Work out the finished part from the listing and answer in its coordinate system (mm). A direction names the side the tool comes from. Round coordinates to 2 decimals unless told otherwise and drop trailing zeros. Loops run counter-clockwise (first coordinate to the right, second up) from the corner with the lowest first, then second, coordinate; pieces in that order, holes last. Notation, with made-up numbers: (30, 35.5) -> (34, 35.5) arc R6 ccw to (34, 40.5) -> close; hole circle Ø10 at (52, 57.5). An arc over 180 degrees is marked (long way). Write item = value, one per line. Start each with the question number.
Autodesk Inventor part; units mm, degrees
ref_plane "YZ Plane" through (0, 0, 0) normal (1, 0, 0) x (0, 1, 0)
ref_plane "XZ Plane" through (0, 0, 0) normal (0, 1, 0) x (-1, 0, 0)
ref_plane "XY Plane" through (0, 0, 0) normal (0, 0, 1) x (1, 0, 0)
sketch "Sketch1" plane through (0, 0, 0) normal (0, 0, 1) x (1, 0, 0)
  line L0 (-6.3366, 6.9163) -> (21.6034, 6.9163)
  line L1 (21.6034, 6.9163) -> (21.6034, -8.3237)
  line L2 (21.6034, -8.3237) -> (-6.3366, -8.3237)
  line L3 (-6.3366, -8.3237) -> (-6.3366, 6.9163)
  point P0 (0, 0)
  dimension "d0" = 27.94
  dimension "d1" = 15.24
extrude "Extrusion1" add sketch "Sketch1" along normal blind 7.62
sketch "Sketch2" plane through (0, 0, 7.62) normal (0, 0, 1) x (1, 0, 0)
  line L0 (-6.3366, 6.9163) -> (-6.3366, -8.3237)
  line L1 (21.6034, -8.3237) -> (21.6034, 6.9163)
  line L2 (21.6034, -0.052) -> (21.6034, 2.361)
  line L3 (-6.3366, 2.361) -> (-6.3366, -0.052)
  line L4 (21.6034, 6.9163) -> (-6.3366, 6.9163)
  line L5 (-6.3366, -8.3237) -> (21.6034, -8.3237)
  line L6 (0.9631, 2.361) -> (-0.2406, 2.361)
  line L7 (-0.2406, -0.052) -> (0.9631, -0.052)
  line L8 (-0.2406, -0.052) -> (-0.2406, 2.361)
  line L9 (-0.2406, -0.052) -> (3.0821, -0.052)
  line L10 (3.0821, -0.052) -> (3.0821, 2.361)
  line L11 (3.0821, 2.361) -> (-0.2406, 2.361)
  line L12 (-0.2406, 2.361) -> (-0.2406, -0.052)
  line L13 (14.3038, 2.361) -> (15.5074, 2.361)
  line L14 (15.5074, -0.052) -> (14.3038, -0.052)
  line L15 (15.5074, -0.052) -> (15.5074, 2.361)
  line L16 (15.5074, -0.052) -> (12.1847, -0.052)
  line L17 (12.1847, -0.052) -> (12.1847, 2.361)
  line L18 (12.1847, 2.361) -> (15.5074, 2.361)
  line L19 (15.5074, 2.361) -> (15.5074, -0.052)
  line L20 (-6.3366, -0.7037) -> (21.6034, -0.7037)
  line L21 (-6.3366, 2.361) -> (21.6034, 2.361)
  line L22 (21.6034, 2.361) -> (21.6034, -0.052)
  line L23 (21.6034, -0.052) -> (-6.3366, -0.052)
  line L24 (-6.3366, -0.052) -> (-6.3366, 2.361)
  point P0 (0, 0)
  point P1 (-0.2406, 1.1545)
  point P2 (15.2669, -0.3643)
  point P3 (15.5074, 1.1545)
  point P4 (15.5074, -0.052)
  point P5 (21.6034, -0.052)
  point P6 (15.5074, 2.361)
  point P7 (-6.3366, -0.052)
  point P8 (-0.2406, -0.052)
  point P9 (-0.2406, 2.361)
  point P10 (-6.3366, 2.361)
  point P11 (3.0821, -0.052)
  point P12 (12.1847, -0.052)
  point P13 (12.1847, 2.361)
  point P14 (3.0821, 2.361)
  dimension "d6" = 6.096
extrude "Extrusion2" add sketch "Sketch2" along normal blind 8.7376 contours L6 L11 L10 L9 L7 L8 | L15 L14 L16 L17 L18 L13
sketch "Sketch3" plane through (-0.2406, 2.361, 7.62) normal (0, 1, 0) x (1, 0, 0)
  line L0 (3.3227, -8.7376) -> (0, -8.7376)
  line L1 (-6.096, 7.62) -> (21.844, 7.62)
  line L2 (3.3227, -11.3552) -> (3.3227, -8.7376)
  line L3 (12.4253, -11.3552) -> (12.4253, -8.7376)
  line L4 (17.2091, -8.255) -> (17.2091, -15.2732)
  line L5 (17.2091, -15.2732) -> (14.9854, -19.057)
  line L6 (14.9854, -19.057) -> (12.4253, -19.057)
  line L7 (12.4253, -19.057) -> (12.4253, -8.7376)
  line L8 (7.874, 7.62) -> (7.874, -24.8322)
  line L9 (3.3227, -11.3552) -> (3.3227, -8.7376)
  line L10 (-1.4611, -8.255) -> (-1.4611, -15.2732)
  line L11 (-1.4611, -15.2732) -> (0.7626, -19.057)
  line L12 (0.7626, -19.057) -> (3.3227, -19.057)
  line L13 (3.3227, -19.057) -> (3.3227, -8.7376)
  line L14 (17.2091, -8.255) -> (12.4253, -8.255)
  line L15 (12.4253, 0) -> (12.4253, -8.7376)
  line L16 (12.4253, -8.255) -> (12.4253, -8.7376)
  line L17 (-1.4611, -8.255) -> (3.3227, -8.255)
  line L18 (3.3227, 0) -> (3.3227, -8.7376)
  line L19 (3.3227, -8.255) -> (3.3227, -8.7376)
  point P0 (0.2406, 7.62)
extrude "Extrusion4" add sketch "Sketch2" along normal blind 25.4 contours L6 L11 L10 L9 L7 L8 | L15 L14 L16 L17 L18 L13
sketch "Sketch4" plane through (-6.3366, 6.9163, 0) normal (0, 1, 0) x (1, 0, 0)
  point P0 (6.3366, 0)
sketch "Sketch5" plane through (0, 0, 7.62) normal (0, 0, 1) x (1, 0, 0)
  line L0 (21.6034, 6.9163) -> (-6.3366, 6.9163)
  line L1 (-6.3366, 15.6735) -> (21.6034, 15.6735)
  line L2 (21.6034, 15.6735) -> (21.6034, 6.9163)
  line L3 (21.6034, 6.9163) -> (-6.3366, 6.9163)
  line L4 (-6.3366, 6.9163) -> (-6.3366, 15.6735)
  point P0 (0, 0)
extrude "Extrusion5" add sketch "Sketch5" along normal blind 17.145 and the other way blind 7.62
extrude "Extrusion6" cut sketch "Sketch2" against normal blind 25.4 contours L20 L1 L5 L0
extrude "Extrusion7" add sketch "Sketch2" along normal blind 4.7625 contours L21 L8 L23 L0 | L1 L23 L15 L21 | L21 L17 L23 L10
extrude "Extrusion8" add sketch "Sketch3" against normal up to surface (2.413 mm away)
sketch "Sketch6" plane through (-6.3366, -0.052, 7.62) normal (0, -1, 0) x (1, 0, 0)
  line L0 (27.94, 0) -> (27.94, 4.7625)
  line L1 (21.844, 4.7625) -> (21.844, 8.255)
  line L2 (27.94, 0) -> (21.844, 0)
  line L3 (21.844, 0) -> (21.844, 4.7625)
  line L4 (21.844, 4.7625) -> (27.94, 4.7625)
  line L5 (27.94, 4.7625) -> (27.94, 0)
  line L6 (18.5213, 4.7625) -> (18.5213, 25.4)
  line L7 (18.5213, 4.7625) -> (9.4187, 4.7625)
  line L8 (9.4187, 4.7625) -> (9.4187, 0)
  line L9 (9.4187, 0) -> (18.5213, 0)
  line L10 (18.5213, 0) -> (18.5213, 4.7625)
  line L11 (6.096, 4.7625) -> (6.096, 8.255)
  line L12 (0, 0) -> (0, 4.7625)
  line L13 (6.096, 4.7625) -> (0, 4.7625)
  line L14 (0, 4.7625) -> (0, 0)
  line L15 (0, 0) -> (6.096, 0)
  line L16 (6.096, 0) -> (6.096, 4.7625)
  point P0 (6.3366, -7.62)
  point P1 (21.844, 8.7376)
  point P2 (18.5213, 19.057)
  point P3 (6.096, 8.7376)
extrude "Extrusion9" cut sketch "Sketch6" against normal up to surface (6.9683 mm away)
sketch "Sketch7" plane through (12.1847, -0.052, 7.62) normal (0, -1, 0) x (1, 0, 0)
  line L0 (3.3227, 17.7594) -> (4.7838, 15.2732)
  line L1 (3.3227, 17.7594) -> (2.3659, 19.3874)
  line L2 (2.3659, 19.3874) -> (2.3659, 25.4)
  line L3 (3.3227, 25.4) -> (0, 25.4)
  line L4 (3.3227, 17.7594) -> (3.3227, 25.4)
  line L5 (2.3659, 25.4) -> (3.3227, 25.4)
  line L6 (3.3227, 25.4) -> (3.3227, 17.7594)
  line L7 (-18.5213, -7.62) -> (9.4187, -7.62)
  line L8 (-12.4253, 17.7594) -> (-11.4685, 19.3874)
  line L9 (-11.4685, 19.3874) -> (-11.4685, 25.4)
  line L10 (-12.4253, 17.7594) -> (-12.4253, 25.4)
  line L11 (-11.4685, 25.4) -> (-12.4253, 25.4)
  line L12 (-12.4253, 25.4) -> (-12.4253, 17.7594)
  line L13 (-12.4253, 8.7376) -> (-13.8865, 8.255)
  line L14 (-9.1825, 8.7376) -> (-9.1026, 8.7376)
  line L15 (-9.1026, 0) -> (-9.1026, 25.4)
  line L16 (-10.6842, 5.3569) -> (-10.764, 0)
  line L17 (-9.1026, 0) -> (-12.4253, 0)
  line L18 (-9.1026, 0) -> (-9.1026, 8.7376)
  line L19 (-10.764, 0) -> (-9.1026, 0)
  line L20 (9.4187, -7.62) -> (-18.5213, -7.62)
  line L21 (-18.5213, 17.145) -> (9.4187, 17.145)
  line L22 (1.5816, 5.3569) -> (1.6613, 0)
  line L23 (1.6613, 0) -> (0, 0)
  line L24 (0, 0) -> (0, 8.7376)
  line L25 (-4.5513, -7.62) -> (-4.5513, 0)
  line L26 (-4.5513, 11.274) -> (-4.5513, 11.3382)
  line L27 (-9.1026, 8.7376) -> (-10.6842, 5.3569)
  line L28 (0, 8.7376) -> (1.5816, 5.3569)
  point P0 (-12.1847, -7.62)
extrude "Extrusion10" cut sketch "Sketch7" against normal up to surface (6.9683 mm away)
fillet "Fillet1" radius 3.175 4 edges at (0.7162, 1.1545, 33.02) (14.5507, 1.1545, 33.02) (16.9686, 1.1545, 22.8932) (-1.7017, 1.1545, 22.8932)
sketch "Sketch8" plane through (-0.2406, -0.052, 7.62) normal (0, -1, 0) x (1, 0, 0)
  arc A0 (-1.0234, 16.018) -> (-1.4611, 14.4093) centre (1.7139, 14.4093) ccw
  line L0 (-1.4611, 8.255) -> (-1.4611, 14.4093)
  line L1 (0, 0) -> (0, 8.255)
  line L2 (1.6613, 0) -> (0, 0)
  line L3 (1.6613, 0) -> (1.7411, 5.3569)
  line L4 (1.7411, 5.3569) -> (3.3227, 8.7376)
  line L5 (3.3227, 8.7376) -> (3.3227, 25.4)
  arc A1 (3.3227, 25.4) -> (0.9568, 22.3298) centre (4.1318, 22.3298) ccw
  line L6 (0.9568, 22.3298) -> (0.9568, 19.3874)
  line L7 (0.9568, 19.3874) -> (-1.0234, 16.018)
  arc A2 (17.2091, 14.4093) -> (16.7714, 16.018) centre (14.0341, 14.4093) ccw
  line L8 (16.7714, 16.018) -> (14.7912, 19.3874)
  line L9 (14.7912, 19.3874) -> (14.7912, 22.3298)
  arc A3 (14.7912, 22.3298) -> (12.4253, 25.4) centre (11.6162, 22.3298) ccw
  line L10 (12.4253, 8.7376) -> (12.4253, 25.4)
  line L11 (12.4253, 8.7376) -> (14.0069, 5.3569)
  line L12 (14.0069, 5.3569) -> (14.0867, 0)
  line L13 (15.748, 0) -> (14.0867, 0)
  line L14 (15.748, 0) -> (15.748, 8.255)
  line L15 (17.2091, 14.4093) -> (17.2091, 8.255)
  line L16 (17.2091, 8.255) -> (15.748, 8.255)
  line L17 (0, 8.255) -> (-1.4611, 8.255)
  point P0 (0.2406, -7.62)
extrude "Extrusion11" add sketch "Sketch8" against normal blind 3.81
sketch "Sketch9" plane through (0, 0, 7.62) normal (0, 0, 1) x (1, 0, 0)
  line L0 (9.6447, 0.3123) -> (5.6221, 0.3123)
  line L1 (5.6221, 0.3123) -> (5.6221, 4.1223)
  line L2 (5.6221, 4.1223) -> (9.6447, 4.1223)
  line L3 (9.6447, 4.1223) -> (9.6447, 0.3123)
  line L4 (12.1847, -0.052) -> (12.1847, 3.758)
  line L5 (3.0821, -0.052) -> (3.0821, 3.758)
  point P0 (0, 0)
  dimension "d30" = 2.54
  dimension "d31" = 2.54
extrude "Extrusion12" add sketch "Sketch9" along normal blind 18.0975
sketch "Sketch10" plane through (21.6034, 6.9163, 24.765) normal (1, 0, 0) x (0, 0, -1)
  line L0 (17.145, 0) -> (0, 0)
  line L1 (24.765, -7.62) -> (17.145, -7.62)
  line L2 (17.145, 0) -> (24.765, 0)
  line L3 (24.765, 0) -> (24.765, -7.62)
  line L4 (24.765, -7.62) -> (17.145, -7.62)
  line L5 (17.145, -7.62) -> (17.145, 0)
  point P0 (24.765, -6.9163)
extrude "Extrusion13" add sketch "Sketch10" along normal blind 6.1214 and the other way blind 34.0614
sketch "Sketch11" plane through (0, 0, 7.62) normal (0, 0, 1) x (1, 0, 0)
  line L0 (21.6034, 15.6735) -> (-6.3366, 15.6735)
  line L1 (9.6447, 0.3123) -> (5.6221, 0.3123)
  line L2 (-12.458, -0.7037) -> (-12.458, 6.9163)
  line L3 (-12.458, -0.7037) -> (27.7248, -0.7037)
  line L4 (-11.1046, -0.7037) -> (-12.458, -0.7037)
  line L5 (-12.458, -0.7037) -> (-12.458, 4.1961)
  line L6 (21.6034, -0.7037) -> (27.7131, -0.7037)
  line L7 (27.7131, -0.7037) -> (27.7131, 4.8182)
  line L8 (27.7131, 4.8182) -> (22.941, 4.8182)
  line L9 (21.6034, 4.8182) -> (21.6034, -0.7037)
  line L10 (-6.3366, -0.7037) -> (-12.4462, -0.7037)
  line L11 (-12.4462, -0.7037) -> (-12.4462, 4.8182)
  line L12 (-12.4462, 4.8182) -> (-7.6742, 4.8182)
  line L13 (-6.3366, 4.8182) -> (-6.3366, -0.7037)
  line L14 (21.6034, 6.9163) -> (27.7248, 6.9163)
  line L15 (22.941, 4.8182) -> (22.941, -0.7037)
  line L16 (7.6334, 0.3123) -> (7.6334, -0.7037)
  line L17 (-7.6742, 4.8182) -> (-7.6742, -0.7037)
  point P0 (0, 0)
  point P1 (22.941, 6.9163)
  point P2 (-7.6742, 6.9163)
  point P3 (-7.6742, -0.7037)
extrude "Extrusion14" add sketch "Sketch11" along normal blind 15.875
properties part number "Attachment6"
Item 1: Section B-B (x = 7.5) is taken. Determine the outline of the cut face in (y, z) (1 decimal), then the cut area to 3 significant figures.
Item 2: Section D-D (y = 11.25) is taken. Determine the outline of the cut face in (x, z) (3 decimals), then the cut area to 3 significant figures.
Item 3: Flat-ended cylindrical pins translate along their axes: pin 1 (9.5 mm diameter, centred on x = 1.5, y = 12.5, fed in from +Z) (3 decimals); pin 2 (1.1 mm diameter, centred on y = 2, z = 11, fed in from +X); pin 3 (4 mm diameter, centred on y = 2, z = 26.5, fed in from +X). Find the tip coordinate at first contact, or state that the pin passes through.
Item 4: Find the intervals of material crossed by line 1 along X through (y, z) = (1, 13); line 2 along Y through (x, z) = (14, 11); line 3 along X through (y, z) = (0, 11), in increasing order. Write a range as [from, to].
Item 5: Section A-A (z = 28) is taken. Determine the outline of the cut face in (x, y).
Item 6: The mould has two halves that part along X. Classify faces 1 (the flat face through (21.603, 11, 12)), 2 (the flat face through (1, -0.052, 20)), 3 (the flat face through (0.716, 2, 28)), 4 (the flat face through (15.507, 2, 12)): pulls with the +X half, pulls with the -X half, needs draft (parallel to the pull), parting line crosses it, or undercut.
Item 7: A tool of negligible diameter and unlimited length cuts with its end or side. For faces 5 (the cylindrical face through (16.86, 3.05, 22.85)), 6 (the flat face through (22.941, 2, 15)), 7 (the flat face through (14, 3.758, 20)), from which of +Z, -Z, +X, -X, +Y, -Y can it reach the whole face along a straight path? Write none if from no direction.
Item 8: Section C-C (z = 12.5) is taken. Determine the outline of the cut face in (x, y).
Worked answers:
q1.outline = (-0.7, 0) -> (15.7, 0) -> (15.7, 24.8) -> (6.9, 24.8) -> (6.9, 7.6) -> (4.1, 7.6) -> (4.1, 25.7) -> (0.3, 25.7) -> (0.3, 7.6) -> (-0.7, 7.6) -> close
q1.area = 344 mm2
q2.outline = (-6.337, 0) -> (21.603, 0) -> (21.603, 24.765) -> (-6.337, 24.765) -> close
q2.area = 692 mm2
q3.pin_1 = 24.765
q3.pin_2 = 27.71
q3.pin_3 = 16.02
q4.line_1 = [-12.45, -7.67], [-0.24, 1.51], [5.62, 9.64], [13.76, 15.51], [22.94, 27.71]
q4.line_2 = [-0.05, 3.76], [6.92, 15.67]
q4.line_3 = [-12.45, -7.67], [-0.24, 1.47], [13.8, 15.51], [22.94, 27.71]
q5.outline = (0.72, -0.05) -> (3.08, -0.05) -> (3.08, 3.76) -> (0.72, 3.76) -> close; (12.18, -0.05) -> (14.55, -0.05) -> (14.55, 3.76) -> (12.18, 3.76) -> close
q6.face_1 = pulls with the +X half
q6.face_2 = undercut
q6.face_3 = pulls with the -X half
q6.face_4 = undercut
q7.face_5 = +Z, -Y
q7.face_6 = +Z, +Y, -Y
q7.face_7 = +Z
q8.outline = (-12.45, -0.7) -> (-7.67, -0.7) -> (-7.67, 4.82) -> (-12.45, 4.82) -> close; (-6.34, 6.92) -> (21.6, 6.92) -> (21.6, 15.67) -> (-6.34, 15.67) -> close; (-0.24, -0.05) -> (1.49, -0.05) -> (1.49, 3.76) -> (-0.24, 3.76) -> close; (5.62, 0.31) -> (9.64, 0.31) -> (9.64, 4.12) -> (5.62, 4.12) -> close; (13.77, -0.05) -> (15.51, -0.05) -> (15.51, 3.76) -> (13.77, 3.76) -> close; (22.94, -0.7) -> (27.71, -0.7) -> (27.71, 4.82) -> (22.94, 4.82) -> close
